Solid Edge part; units mm, degrees
sketch "Sketch1" plane through (0, 0, 0) normal (0, 0, 1) x (1, 0, 0)
  line L0 (-175, 60) -> (-175, -60)
  line L1 (-175, -60) -> (-100, -75)
  line L2 (-100, -75) -> (100, -75)
  line L3 (100, -75) -> (175, -60)
  line L4 (175, -60) -> (175, 60)
  line L5 (175, 60) -> (100, 75)
  line L6 (100, 75) -> (-100, 75)
  line L7 (-100, 75) -> (-175, 60)
  circle A0 centre (0, 0) radius 30
  dimension "D1" = 175
  dimension "D2" = 100
  dimension "D3" = 175
extrude "Protrusion1" add sketch "Sketch1" along normal blind 40
sketch "Sketch2" plane through (0, 0, 40) normal (0, 0, 1) x (1, 0, 0)
  line L0 (-160, 0) -> (-160, 63)
  line L1 (-160, 63) -> (-130, 69)
  line L2 (-130, 0) -> (-130, 69)
  arc A0 (-130, 0) -> (-160, 0) centre (-145, 0) cw
extrude "ExtrudedCutout_1" cut sketch "Sketch2" against normal blind 266.7716
mirror "Mirror1" about plane through (0, 0, 0) normal (1, 0, 0) of "ExtrudedCutout_1"
Read the model definition and answer for the solid it produces. Units are mm, in the model's axes. A direction names the side the tool comes from. Coordinates: 2 decimals unless noted, no trailing zeros. Loops run counter-clockwise (first coordinate to the right, second up) from the corner with the lowest first, then second, coordinate; pieces in that order, holes last.
Q1. The mould has two halves that part along Y. Classify faces 3 (the face through (-29.97, -1.32, 19.72)), 4 (the face through (145, -15, 20)), 5 (the face through (-138, -67.4, 19.7)): +Y half, -Y half, draft (parallel to the pull), parting line (faces both ways), or undercut.
Q2. The part is cut by section D-D on y = -10.5. Write down the section's boundary in (x, z), and give its area (3 significant figures).
Q3. The part is cut by section C-C on y = 25. Write down the section's boundary in (x, z).
Q4. Which of the six approach directions +Z, -Z, +X, -X, +Y, -Y give full straight-line access (tool end or side, diameter ignored) to faces 1 (the face through (-167.4, 61.52, 19.72)), 2 (the face through (-160, 31, 20))?
Q5. The part is cut by section B-B on x = 0. Write down the section's boundary in (y, z).
Q6. The part is cut by section A-A on z = 32. Write down the section's boundary in (x, y), and give its area (3 significant figures).
Q7. Consider probe 1 along X at (y, z) = (34, 24); probe 2 along X at (y, z) = (-6, 19); probe 3 along X at (y, z) = (3.5, 30). Determine where each line is inside the solid, lowest interval first.
Results below:
1. face 3: undercut
1. face 4: +Y half
1. face 5: -Y half
2. outline: (-175, 0) - (-155.71, 0) - (-155.71, 40) - (-175, 40) - close; (-134.29, 0) - (-28.1, 0) - (-28.1, 40) - (-134.29, 40) - close; (28.1, 0) - (134.29, 0) - (134.29, 40) - (28.1, 40) - close; (155.71, 0) - (175, 0) - (175, 40) - (155.71, 40) - close
2. area: 10,000 mm2
3. outline: (-175, 0) - (-160, 0) - (-160, 40) - (-175, 40) - close; (-130, 0) - (-16.58, 0) - (-16.58, 40) - (-130, 40) - close; (16.58, 0) - (130, 0) - (130, 40) - (16.58, 40) - close; (160, 0) - (175, 0) - (175, 40) - (160, 40) - close
4. face 1: +Z, -Z, -X, +Y
4. face 2: +Z, -Z, +Y
5. outline: (-75, 0) - (-30, 0) - (-30, 40) - (-75, 40) - close; (30, 0) - (75, 0) - (75, 40) - (30, 40) - close
6. outline: (-175, -60) - (-100, -75) - (100, -75) - (175, -60) - (175, 60) - (160, 63) - (160, 0) arc R15 cw to (130, 0) - (130, 69) - (100, 75) - (-100, 75) - (-130, 69) - (-130, 0) arc R15 cw to (-160, 0) - (-160, 63) - (-175, 60) - close; hole circle Ø60 at (0, 0)
6. area: 42,800 mm2
7. probe 1: x = -175 to -160, -130 to 130, 160 to 175
7. probe 2: x = -175 to -158.75, -131.25 to -29.39, 29.39 to 131.25, 158.75 to 175
7. probe 3: x = -175 to -160, -130 to -29.8, 29.8 to 130, 160 to 175
